Check sheet for the modelled part. Datum: model origin and axes. Units: mm. A direction names the side the tool comes from. Round coordinates to 2 decimals unless told otherwise and drop trailing zeros. Write each loop counter-clockwise with the first axis right and the second up, starting at its lowest first coordinate (ties: lowest second). Pieces come first, ordered by that corner, then holes. Notation, with made-up numbers: (33, 58) -> (90, 58) arc R25 ccw to (90, 80) -> close; hole circle Ø1 at (-7, 57.25). An arc over 180 degrees is marked (long way). One line per item, written item: value.
from build123d import *

# Parameters (mm, degrees)
F0_W           = 53
F0_H           = 66
F1_DEPTH       = 12.5
F2_W           = 64
F2_H           = 8.5
F3_DEPTH       = 52
F4_W           = 46
F4_H           = 35
F5_DEPTH       = 5
F6_W           = 14
F6_H           = 12.5
F7_DEPTH       = 1
F8_W           = 14
F8_H           = 14
F9_DEPTH       = 14.1
F11_DEPTH      = 14
F12_W          = 14
F12_H          = 14
F13_DEPTH      = 1
F13_DEPTH_BACK = 13.1
F15_DEPTH      = 14
F16_W          = 5
F16_H          = 4
F17_DEPTH      = 13.1
F18_W          = 5
F18_H          = 4
F19_DEPTH      = 13.1
F20_W          = 66
F20_H          = 4
F21_DEPTH      = 6
F22_W          = 10
F22_H          = 4.5
F23_DEPTH      = 0.5
F23_DEPTH_BACK = 3.5
F25_DEPTH      = 10
F26_W          = 10
F26_H          = 12.5
F27_DEPTH      = 4
F29_DEPTH      = 10
F30_W          = 10
F30_H          = 4.5
F31_DEPTH      = 0.5
F31_DEPTH_BACK = 3.5
F33_DEPTH      = 10
F34_W          = 10
F34_H          = 12.5
F35_DEPTH      = 4
F37_DEPTH      = 10
F39_DEPTH      = 2.5
F40_R          = 1.5
F41_DEPTH      = 6
F43_DEPTH      = 2.5
F44_R          = 1.5
F45_DEPTH      = 6
F46_R          = 1.7
F47_DEPTH      = 5
F49_DEPTH      = 2.5
F50_R          = 1.7
F51_DEPTH      = 6


with BuildPart() as f1:
    # F0 (on Top) → F1 (new body)
    with BuildSketch(Plane.XY):
        Rectangle(F0_W, F0_H)
    extrude(amount=F1_DEPTH)

    # F2 (on face) → F3 (cut)
    with BuildSketch(Plane(origin=(-26.5, 0, 0), x_dir=(0, -1, 0), z_dir=(-1, 0, 0))):
        with Locations((0, 8.25)):
            Rectangle(F2_W, F2_H)
    extrude(amount=-F3_DEPTH, mode=Mode.SUBTRACT)

    # F4 (on face) → F5 (cut)
    with BuildSketch(Plane.XY.offset(4)):
        with Locations((-0.5, 0)):
            Rectangle(F4_W, F4_H)
    extrude(amount=-F5_DEPTH, mode=Mode.SUBTRACT)

    # F6 (on face) → F7 (cut)
    with BuildSketch(Plane.YZ.offset(26.5)):
        with Locations((-21, 6.25)):
            Rectangle(F6_W, F6_H)
    extrude(amount=-F7_DEPTH, mode=Mode.SUBTRACT)

    # F8 (on face) → F9 (join)
    with BuildSketch(Plane.YZ.offset(25.5)):
        with Locations((-21, 7)):
            Rectangle(F8_W, F8_H)
    extrude(amount=F9_DEPTH)

    # F10 (on face) → F11 (cut)
    with BuildSketch(Plane.XZ.offset(28)):
        with BuildLine():
            Line((27.8857629746, 14), (27.8857629746, 12.911010872))
            ThreePointArc((27.8857629746, 12.911010872), (26.5594651822, 8.159449016), (29.2118961029, 4))
            Line((29.2118961029, 4), (35.8752286024, 4))
            ThreePointArc((35.8752286024, 4), (38.5276595231, 8.159449016), (37.2013617307, 12.911010872))
            Line((37.2013617307, 12.911010872), (37.2013617307, 14))
            Line((37.2013617307, 14), (27.8857629746, 14))
        make_face()
    extrude(amount=-F11_DEPTH, mode=Mode.SUBTRACT)

    # F12 (on face) → F13 (join, two sides)
    with BuildSketch(Plane.YZ.offset(26.5)) as f13_sk:
        with Locations((21, 7)):
            Rectangle(F12_W, F12_H)
    extrude(amount=-F13_DEPTH)
    extrude(f13_sk.sketch, amount=F13_DEPTH_BACK)

    # F14 (on face) → F15 (cut)
    with BuildSketch(Plane(origin=(0, 28, 0), x_dir=(-1, 0, 0), z_dir=(0, 1, 0))):
        with BuildLine():
            Line((-37.3720750213, 14), (-37.3720750213, 12.935615631))
            ThreePointArc((-37.3720750213, 12.935615631), (-38.7212150513, 8.175292403), (-36.0664477535, 4))
            Line((-36.0664477535, 4), (-29.4031152539, 4))
            ThreePointArc((-29.4031152539, 4), (-26.7483479561, 8.175292403), (-28.0974879861, 12.935615631))
            Line((-28.0974879861, 12.935615631), (-28.0974879861, 14))
            Line((-28.0974879861, 14), (-37.3720750213, 14))
        make_face()
    extrude(amount=-F15_DEPTH, mode=Mode.SUBTRACT)

    # F16 (on face) → F17 (join, through all)
    with BuildSketch(Plane.YZ.offset(26.5)):
        with Locations((-30.5, 2)):
            Rectangle(F16_W, F16_H)
    extrude(amount=F17_DEPTH)

    # F18 (on face) → F19 (join, through all)
    with BuildSketch(Plane.YZ.offset(26.5)):
        with Locations((30.5, 2)):
            Rectangle(F18_W, F18_H)
    extrude(amount=F19_DEPTH)

    # F20 (on face) → F21 (join)
    with BuildSketch(Plane.YZ.offset(39.6)):
        with Locations((0, 2)):
            Rectangle(F20_W, F20_H)
    extrude(amount=F21_DEPTH)

    # F22 (on face) → F23 (join, two sides)
    with BuildSketch(Plane.XZ.offset(33)) as f23_sk:
        with Locations((32.55, 2.25)):
            Rectangle(F22_W, F22_H)
    extrude(amount=-F23_DEPTH)
    extrude(f23_sk.sketch, amount=F23_DEPTH_BACK)

    # F24 (on face) → F25 (cut)
    with BuildSketch(Plane.YZ.offset(37.55)):
        Polygon((-36.5, 0), (-33, 0), (-36.5, 3.5), align=None)
    extrude(amount=-F25_DEPTH, mode=Mode.SUBTRACT)

    # F26 (on face) → F27 (join)
    with BuildSketch(Plane.XZ.offset(33)):
        with Locations((-15.45, 6.25)):
            Rectangle(F26_W, F26_H)
    extrude(amount=F27_DEPTH)

    # F28 (on face) → F29 (cut, through all)
    with BuildSketch(Plane(origin=(-20.45, 0, 0), x_dir=(0, -1, 0), z_dir=(-1, 0, 0))):
        Polygon((33, 0), (37, 0), (37, 4.0411888622), align=None)
    extrude(amount=-F29_DEPTH, mode=Mode.SUBTRACT)

    # F30 (on face) → F31 (join, two sides)
    with BuildSketch(Plane(origin=(0, 33, 0), x_dir=(-1, 0, 0), z_dir=(0, 1, 0))) as f31_sk:
        with Locations((-32.55, 2.25)):
            Rectangle(F30_W, F30_H)
    extrude(amount=-F31_DEPTH)
    extrude(f31_sk.sketch, amount=F31_DEPTH_BACK)

    # F32 (on face) → F33 (cut, through all)
    with BuildSketch(Plane.YZ.offset(37.55)):
        Polygon((36.5, 3.5), (33, 0), (36.5, 0), align=None)
    extrude(amount=-F33_DEPTH, mode=Mode.SUBTRACT)

    # F34 (on face) → F35 (join)
    with BuildSketch(Plane(origin=(0, 33, 0), x_dir=(-1, 0, 0), z_dir=(0, 1, 0))):
        with Locations((15.45, 6.25)):
            Rectangle(F34_W, F34_H)
    extrude(amount=F35_DEPTH)

    # F36 (on face) → F37 (cut, through all)
    with BuildSketch(Plane.YZ.offset(-10.45)):
        Polygon((37, 4), (33, 0), (37, 0), align=None)
    extrude(amount=-F37_DEPTH, mode=Mode.SUBTRACT)

    # F38 (on face) → F39 (cut)
    with BuildSketch(Plane(origin=(0, -32, 0), x_dir=(-1, 0, 0), z_dir=(0, 1, 0))):
        Polygon((15.5747217333, 12.2), (12.7910795745, 10.6214096491), (12.7663578412, 7.4214096491), (15.5252782667, 5.8), (18.3089204255, 7.3785903509), (18.3336421588, 10.5785903509), align=None)
    extrude(amount=-F39_DEPTH, mode=Mode.SUBTRACT)

    # F40 (on face) → F41 (cut)
    with BuildSketch(Plane(origin=(0, -32, 0), x_dir=(-1, 0, 0), z_dir=(0, 1, 0))):
        with Locations((15.55, 9)):
            Circle(F40_R)
    extrude(amount=-F41_DEPTH, mode=Mode.SUBTRACT)

    # F42 (on face) → F43 (cut)
    with BuildSketch(Plane.XZ.offset(-32)):
        Polygon((-15.6680351614, 5.8), (-12.8377362886, 7.2977785517), (-12.7197011272, 10.4977785517), (-15.4319648386, 12.2), (-18.2622637114, 10.7022214483), (-18.3802988728, 7.5022214483), align=None)
    extrude(amount=-F43_DEPTH, mode=Mode.SUBTRACT)

    # F44 (on face) → F45 (cut)
    with BuildSketch(Plane.XZ.offset(-32)):
        with Locations((-15.55, 9)):
            Circle(F44_R)
    extrude(amount=-F45_DEPTH, mode=Mode.SUBTRACT)

    # F46 (on face) → F47 (cut)
    with BuildSketch(Plane.XY.offset(4)):
        with Locations((42.6, -25)):
            Circle(F46_R)
        with Locations((42.6, -9)):
            Circle(F46_R)
        with Locations((42.6, 9)):
            Circle(F46_R)
        with Locations((42.6, 25)):
            Circle(F46_R)
    extrude(amount=-F47_DEPTH, mode=Mode.SUBTRACT)

    # F48 (on face) → F49 (cut)
    with BuildSketch(Plane.XY.offset(4)):
        Polygon((-12.9739972428, 21.55), (-10.2157173293, 23.1725190483), (-10.2417200865, 26.3725190483), (-13.0260027572, 27.95), (-15.7842826707, 26.3274809517), (-15.7582799135, 23.1274809517), align=None)
        Polygon((2.0260027572, 21.55), (4.7842826707, 23.1725190483), (4.7582799135, 26.3725190483), (1.9739972428, 27.95), (-0.7842826707, 26.3274809517), (-0.7582799135, 23.1274809517), align=None)
        Polygon((17.0260027572, 21.55), (19.7842826707, 23.1725190483), (19.7582799135, 26.3725190483), (16.9739972428, 27.95), (14.2157173293, 26.3274809517), (14.2417200865, 23.1274809517), align=None)
        Polygon((-12.8728363868, -27.95), (-10.1651369013, -26.2398730805), (-10.2923005145, -23.0398730805), (-13.1271636132, -21.55), (-15.8348630987, -23.2601269195), (-15.7076994855, -26.4601269195), align=None)
        Polygon((2.1271636132, -27.95), (4.8348630987, -26.2398730805), (4.7076994855, -23.0398730805), (1.8728363868, -21.55), (-0.8348630987, -23.2601269195), (-0.7076994855, -26.4601269195), align=None)
        Polygon((17.1271636132, -27.95), (19.8348630987, -26.2398730805), (19.7076994855, -23.0398730805), (16.8728363868, -21.55), (14.1651369013, -23.2601269195), (14.2923005145, -26.4601269195), align=None)
    extrude(amount=-F49_DEPTH, mode=Mode.SUBTRACT)

    # F50 (on face) → F51 (cut)
    with BuildSketch(Plane.XY.offset(4)):
        with Locations((-12.9739972428, 24.7725190483)):
            Circle(F50_R)
        with Locations((2.0260027572, 24.7725190483)):
            Circle(F50_R)
        with Locations((17.0260027572, 24.7725190483)):
            Circle(F50_R)
        with Locations((17.1271636132, -24.6398730805)):
            Circle(F50_R)
        with Locations((2.1271636132, -24.6398730805)):
            Circle(F50_R)
        with Locations((-12.8728363868, -24.6398730805)):
            Circle(F50_R)
    extrude(amount=-F51_DEPTH, mode=Mode.SUBTRACT)


solid = f1.part
Item 1: Sectioned sample at C-C on x = 42.6. Enter the section's corners in (y, z), and give its area (3 significant figures).
Answer:
outline: (-33, 0) -> (-26.7, 0) -> (-26.7, 4) -> (-33, 4) -> close; (-23.3, 0) -> (-10.7, 0) -> (-10.7, 4) -> (-23.3, 4) -> close; (-7.3, 0) -> (7.3, 0) -> (7.3, 4) -> (-7.3, 4) -> close; (10.7, 0) -> (23.3, 0) -> (23.3, 4) -> (10.7, 4) -> close; (26.7, 0) -> (33, 0) -> (33, 4) -> (26.7, 4) -> close
area: 210 mm^2
Item 2: Mould release check, pull along Z, two halves, no side actions. Record for faces 4 (the flat face through (-1, 32, 8)), 5 (the flat face through (-24, 0, 4)), 6 (the cylindrical face through (38.517, -21.098, 8.089)): pulls with the +Z half, pulls with the -Z half, needs draft (parallel to the pull), parting line crosses it, or undercut.
Answer:
face 4: needs draft
face 5: pulls with the +Z half
face 6: undercut
Item 3: Tool access check on faces 1 (the flat face through (-16.97, -33.23, 11.38)), 2 (the flat face through (-11.54, -27.11, 2.77)), 3 (the flat face through (26.5, 0, 6)). Record the directions out of +Z, -Z, +X, -X, +Y, -Y that give a thin tool (end or side, any length) a straight path to the whole face; none if there is none.
Answer:
face 1: none
face 2: +Z
face 3: +Z, -Z
Item 4: Thickness scan on line 1 (X direction, y = -3, z = 2); line 2 (Y direction, x = -20.5, z = 6.75); line 3 (Y direction, x = 42.6, z = 1.3). Record the ranges inside material, lowest first.
Answer:
line 1: x = -26.5 to -23.5, 22.5 to 26.5, 39.6 to 45.6
line 2: y = -33 to -32, 32 to 33
line 3: y = -33 to -26.7, -23.3 to -10.7, -7.3 to 7.3, 10.7 to 23.3, 26.7 to 33
Item 5: Sectioned sample at B-B on y = -9. Enter the section's corners in (x, z).
Answer:
outline: (-26.5, 0) -> (-23.5, 0) -> (-23.5, 4) -> (-26.5, 4) -> close; (22.5, 0) -> (26.5, 0) -> (26.5, 12.5) -> (25.5, 12.5) -> (25.5, 4) -> (22.5, 4) -> close; (39.6, 0) -> (40.9, 0) -> (40.9, 4) -> (39.6, 4) -> close; (44.3, 0) -> (45.6, 0) -> (45.6, 4) -> (44.3, 4) -> close
Item 6: Sectioned sample at A-A on x = -2. Enter the section's corners in (y, z).
Answer:
outline: (-33, 0) -> (-17.5, 0) -> (-17.5, 4) -> (-32, 4) -> (-32, 12.5) -> (-33, 12.5) -> close; (17.5, 0) -> (33, 0) -> (33, 12.5) -> (32, 12.5) -> (32, 4) -> (17.5, 4) -> close
Item 7: Depth check by flat-ended pin: P1, Ø2.5, axis at y = -30, z = 9, coming from the +X side; P2, Ø4.5, axis at x = 7.5, y = 30.5, coming from the +Z side; P3, Ø2, axis at y = 17.5, z = 6, coming from the +X side. Enter the tip coordinate at first touch or a pass-through.
Answer:
P1: stops at x = 26.5
P2: stops at z = 12.5
P3: stops at x = 39.6
Item 8: Sectioned sample at D-D on x = 23.5. Enter the section's corners in (y, z).
Answer:
outline: (-33, 0) -> (33, 0) -> (33, 12.5) -> (32, 12.5) -> (32, 4) -> (-32, 4) -> (-32, 12.5) -> (-33, 12.5) -> close
